Verification items for the finished model (mm, model axes). A direction names the side the tool comes from. Give positions to 0.01 mm unless a question says otherwise; leave off trailing zeros. Write each loop counter-clockwise with the first axis right and the second up, starting at its lowest first coordinate (ties: lowest second). Pieces come first, ordered by that corner, then holes. Notation, with made-up numbers: (-36.5, 32.25) - (14.5, 32.25) arc R18 ccw to (14.5, 57.25) - close; hole circle Ø1 at (14, 12). An arc over 180 degrees is marked (long way). Answer as a JSON object with one key per item and string values. Group by question number.
Item 1: Go/stop test with flat-tipped pins: pin 1 (2 mm diameter, centred on y = 1.5, z = 10.5, fed in from +X); pin 2 (1.5 mm diameter, centred on x = -24.5, z = -5, fed in from -Y); pin 3 (2 mm diameter, centred on y = 3.5, z = 10, fed in from +X). Record where each tip stops, or that it passes through.
Item 2: Tool access check on faces 1 (the face through (10.755, 4, -1)), 2 (the face through (-11, 1, -11.637)), 3 (the face through (-5, 0, -26)). Record the directions out of +Z, -Z, +X, -X, +Y, -Y that give a thin tool (end or side, any length) a straight path to the whole face; none if there is none.
Item 3: Sectioned sample at B-B, the plane x = -2.5. Record the boundary of the cut face in (y, z).
Item 4: Sectioned sample at C-C, the plane y = 0.75. Count the separate pieces of the cut face and the enclosed holes in it, and give its area (3 significant figures).
Item 5: Sectioned sample at D-D, the plane x = 9.5. Record the boundary of the cut face in (y, z), and give its area (3 significant figures).
Item 6: Scan lines: line 1 along X through (y, z) = (3.3, 7); line 2 along Z through (x, y) = (-4, 2.25); line 3 along X through (y, z) = (1.4, -9.5). Record each from-to range of solid material in increasing order. Write a range as [from, to].
Item 7: Sectioned sample at A-A, the plane z = -9.5. Record the boundary of the cut face in (x, y), and give its area (3 significant figures).
Item 8: Draft check along X on faces 4 (the face through (-10.955, 1, 10)), 5 (the face through (-5, 0, -12)). Enter one of: +X half, -X half, draft (parallel to the pull), parting line (faces both ways), or undercut.
```python
from build123d import *
from build123d.topology import SkipClean

# Parameters (mm, degrees)
BOSS_EXTRUDE1_DEPTH = 2.54
SKETCH3_W           = 32.640662211
SKETCH3_H           = 18.538410016
BOSS_EXTRUDE3_DEPTH = 2.54
BOSS_EXTRUDE5_START = 0.508
BOSS_EXTRUDE5_DEPTH = 0.508


with BuildPart() as part:
    # Sketch1 → Boss-Extrude1 (new body)
    with BuildSketch(Plane(origin=(0, 0, 0), x_dir=(1, 0, 0), z_dir=(0, 1, 0))):
        with BuildLine():
            ThreePointArc((-39.649349134, 1.286034678), (-38.429647834, -15.641923347), (-21.52975616, -14.08080337))
            Line((-21.52975616, -14.08080337), (12.321775162, -14.079871626))
            ThreePointArc((12.321775162, -14.079871626), (29.221293553, -15.641366687), (30.440421584, 1.286294566))
            ThreePointArc((30.440421584, 1.286294566), (29.220717841, 18.214253603), (12.320825474, 16.653128255))
            Line((12.320825474, 16.653128255), (8.095060057, 16.653011943))
            ThreePointArc((8.095060057, 16.653011943), (-4.605289499, 29.352662378), (-17.304939934, 16.652312823))
            Line((-17.304939934, 16.652312823), (-21.530705351, 16.652196511))
            ThreePointArc((-21.530705351, 16.652196511), (-38.430218697, 18.213690635), (-39.649349134, 1.286034678))
        make_face()
        with BuildLine():
            Line((4.285060058, 16.652907075), (-13.494939935, 16.652417691))
            ThreePointArc((-13.494939935, 16.652417691), (-4.605184631, 25.54266238), (4.285060058, 16.652907075))
        make_face(mode=Mode.SUBTRACT)
        with BuildLine():
            Line((-4.604964725, 11.637139843), (-4.604964725, 14.112662381))
            Line((-4.604964725, 14.112662381), (13.620033749, 14.113164014))
            ThreePointArc((13.620033749, 14.113164014), (28.108622145, 15.790575731), (26.57403613, 1.28616435))
            ThreePointArc((26.57403613, 1.28616435), (28.109123124, -13.217754754), (13.6210332, -11.539835864))
            Line((13.6210332, -11.539835864), (12.321775162, -11.539871625))
            Line((12.321775162, -11.539871625), (12.321775162, -9.03008529))
            Line((12.321775162, -9.03008529), (1.640510114, -9.03008529))
            Line((1.640510114, -9.03008529), (1.640510114, -11.540165621))
            Line((1.640510114, -11.540165621), (-10.954952329, -11.540512304))
            Line((-10.954952329, -11.540512304), (-10.954952329, -9.03008529))
            Line((-10.954952329, -9.03008529), (-21.52975616, -9.03008529))
            Line((-21.52975616, -9.03008529), (-21.52975616, -11.540803369))
            Line((-21.52975616, -11.540803369), (-22.828963748, -11.540839129))
            ThreePointArc((-22.828963748, -11.540839129), (-22.947503255, -11.725155299), (-23.070333709, -11.906640133))
            Line((-23.070333709, -11.906640133), (-23.070333709, -12.058667845))
            Line((-23.070333709, -12.058667845), (-23.177995711, -12.058508621))
            ThreePointArc((-23.177995711, -12.058508621), (-37.535703997, -12.994889522), (-35.782964221, 1.28616435))
            ThreePointArc((-35.782964221, 1.28616435), (-35.926521617, 1.379963865), (-36.0683329, 1.476382925))
            ThreePointArc((-36.0683329, 1.476382925), (-37.19509177, 15.909614485), (-22.829963199, 14.112160749))
            Line((-22.829963199, 14.112160749), (-17.304939934, 14.112312822))
            Line((-17.304939934, 14.112312822), (-17.304939934, 11.637139843))
            Line((-17.304939934, 11.637139843), (-4.604964725, 11.637139843))
        make_face(mode=Mode.SUBTRACT)
    extrude(amount=BOSS_EXTRUDE1_DEPTH)

    # Sketch3 → Boss-Extrude3 (add)
    with BuildSketch(Plane(origin=(0, 2.54, 0), x_dir=(1, 0, 0), z_dir=(0, 1, 0))):
        with BuildLine():
            Line((12.320825474, 16.653128255), (8.095060057, 16.653011943))
            ThreePointArc((8.095060057, 16.653011943), (-4.605289499, 29.352662378), (-17.304939934, 16.652312823))
            Line((-17.304939934, 16.652312823), (-21.530705351, 16.652196511))
            ThreePointArc((-21.530705351, 16.652196511), (-38.430218697, 18.213690635), (-39.649349134, 1.286034678))
            ThreePointArc((-39.649349134, 1.286034678), (-38.429647834, -15.641923347), (-21.52975616, -14.08080337))
            Line((-21.52975616, -14.08080337), (12.321775162, -14.079871626))
            ThreePointArc((12.321775162, -14.079871626), (29.221293553, -15.641366687), (30.440421584, 1.286294566))
            ThreePointArc((30.440421584, 1.286294566), (29.220717841, 18.214253603), (12.320825474, 16.653128255))
        make_face()
        with BuildLine():
            Line((-13.494939935, 16.652417691), (4.285060058, 16.652907075))
            ThreePointArc((4.285060058, 16.652907075), (-4.605184631, 25.54266238), (-13.494939935, 16.652417691))
        make_face(mode=Mode.SUBTRACT)
        with Locations((-5.565360914, 1.202786927)):
            Rectangle(SKETCH3_W, SKETCH3_H, mode=Mode.SUBTRACT)
    extrude(amount=BOSS_EXTRUDE3_DEPTH)

    # Sketch4 → Boss-Extrude5 (add)
    with SkipClean():  # the faces are left unmerged after this step: merging them gives an invalid solid
        with BuildSketch(Plane.XZ.offset(BOSS_EXTRUDE5_START)):
            with BuildLine():
                Line((4.285060058, -16.652907075), (8.095060057, -16.653011943))
                Line((8.095060057, -16.653011943), (12.320825474, -16.653128255))
                ThreePointArc((12.320825474, -16.653128255), (29.220717841, -18.214253603), (30.440421584, -1.286294566))
                ThreePointArc((30.440421584, -1.286294566), (29.221293553, 15.641366687), (12.321775162, 14.079871626))
                Line((12.321775162, 14.079871626), (-21.52975616, 14.08080337))
                ThreePointArc((-21.52975616, 14.08080337), (-38.429647834, 15.641923347), (-39.649349134, -1.286034678))
                ThreePointArc((-39.649349134, -1.286034678), (-38.430218697, -18.213690635), (-21.530705351, -16.652196511))
                Line((-21.530705351, -16.652196511), (-17.304939934, -16.652312823))
                Line((-17.304939934, -16.652312823), (-13.494939935, -16.652417691))
                Line((-13.494939935, -16.652417691), (4.285060058, -16.652907075))
            make_face()
            with BuildLine():
                Line((-22.552623375, 12.048831523), (13.344678341, 12.04784347))
                ThreePointArc((13.344678341, 12.04784347), (28.299197198, 13.740578889), (27.463139128, -1.286197025))
                ThreePointArc((27.463139128, -1.286197025), (28.298681008, -16.313414565), (13.343693226, -14.621156408))
                Line((13.343693226, -14.621156408), (8.095115986, -14.621011944))
                Line((8.095115986, -14.621011944), (-17.304884004, -14.620312824))
                Line((-17.304884004, -14.620312824), (-22.553608377, -14.620168355))
                ThreePointArc((-22.553608377, -14.620168355), (-37.508122345, -16.31290289), (-36.672067047, -1.286131788))
                ThreePointArc((-36.672067047, -1.286131788), (-37.507610583, 13.741084507), (-22.552623375, 12.048831523))
            make_face(mode=Mode.SUBTRACT)
        extrude(amount=-BOSS_EXTRUDE5_DEPTH)


solid = part.part
```
Geometry check:
{
 "1": {"pin 1": "x = 33.05", "pin 2": "y = 2.54", "pin 3": "x = 33.17"},
 "2": {"face 1": "+Y, -Y", "face 2": "-Y", "face 3": "-Z, -Y"},
 "3": {"outline": "(-0.51, -16.65) - (5.08, -16.65) - (5.08, -10.47) - (2.54, -10.47) - (2.54, -14.11) - (0, -14.11) - (0, -14.62) - (-0.51, -14.62) - close; (-0.51, 12.05) - (0, 12.05) - (0, 11.54) - (2.54, 11.54) - (2.54, 8.07) - (5.08, 8.07) - (5.08, 14.08) - (-0.51, 14.08) - close; (0, -29.18) - (5.08, -29.18) - (5.08, -25.29) - (0, -25.29) - close"},
 "4": {"separate pieces": "1", "enclosed holes": "2", "area": "754 mm^2"},
 "5": {"outline": "(-0.51, -16.65) - (5.08, -16.65) - (5.08, -10.47) - (2.54, -10.47) - (2.54, -14.11) - (0, -14.11) - (0, -14.62) - (-0.51, -14.62) - close; (-0.51, 12.05) - (0, 12.05) - (0, 9.03) - (2.54, 9.03) - (2.54, 8.07) - (5.08, 8.07) - (5.08, 14.08) - (-0.51, 14.08) - close", "area": "52.3 mm^2"},
 "6": {"line 1": "[-42.62, -21.89], [10.75, 33.41]", "line 2": "[-29.34, -25.52], [-16.65, -14.11], [11.54, 14.08]", "line 3": "[-42.62, -40.08], [30.87, 33.41]"},
 "7": {"outline": "(-42.62, -0.51) - (-40.59, -0.51) - (-40.59, 0) - (-40.08, 0) - (-40.08, 2.54) - (-21.89, 2.54) - (-21.89, 5.08) - (-42.62, 5.08) - close; (10.75, 2.54) - (30.87, 2.54) - (30.87, 0) - (31.38, 0) - (31.38, -0.51) - (33.41, -0.51) - (33.41, 5.08) - (10.75, 5.08) - close", "area": "125 mm^2"},
 "8": {"face 4": "undercut", "face 5": "undercut"}
}
